from build123d import *

# Parameters (mm, degrees)
BOSS_EXTRUDE1_DEPTH            = 10
SKETCH2_W                      = 12
SKETCH2_H                      = 12.25
BOSS_EXTRUDE2_DEPTH            = 23
SKETCH4_W                      = 65
SKETCH4_H                      = 38.636969104
BOSS_EXTRUDE3_DEPTH            = 10
F_3_6_3_6_DIAMETER_HOLE1_D     = 3.6
F_3_6_3_6_DIAMETER_HOLE1_DEPTH = 10
F_3_6_3_6_DIAMETER_HOLE1_TIP   = 1.081549114
SKETCH21_W                     = 41
SKETCH21_H                     = 12.25
BOSS_EXTRUDE4_DEPTH            = 33
SKETCH23_W                     = 65
SKETCH23_H                     = 43
BOSS_EXTRUDE6_DEPTH            = 14
FILLET1_R                      = 1
F_6_6_6_6_DIAMETER_HOLE1_D     = 6.6
SKETCH28_R                     = 1.8
CUT_EXTRUDE1_DEPTH             = 44.0000001


with BuildPart() as part:
    # Sketch1 → Boss-Extrude1 (new body)
    with BuildSketch(Plane.XY):
        with BuildLine():
            Line((-6, 14.302325581), (-6, -20.697674419))
            Line((-6, -20.697674419), (6, -20.697674419))
            Line((6, -20.697674419), (6, 14.302325581))
            add(Edge.make_bspline(
                [(6, 14.302325581), (6, 18.078005618), (0, 18.078005618), (-6, 18.078005618), (-6, 14.302325581)],
                knots=[0, 0, 0, 1.570796327, 1.570796327, 3.141592654, 3.141592654, 3.141592654], degree=2, weights=[1, 0.707106781, 1, 0.707106781, 1]))
        make_face()
    boss_extrude1 = extrude(amount=BOSS_EXTRUDE1_DEPTH)

    # Sketch2 → Boss-Extrude2 (add)
    with BuildSketch(Plane.XY.offset(10)):
        with Locations((0, -14.572674419)):
            Rectangle(SKETCH2_W, SKETCH2_H)
    boss_extrude2 = extrude(amount=BOSS_EXTRUDE2_DEPTH)

    # Sketch4 → Boss-Extrude3 (add)
    with BuildSketch(Plane.XY.offset(33)):
        with Locations((-26.5, -1.379189867)):
            Rectangle(SKETCH4_W, SKETCH4_H)
    extrude(amount=BOSS_EXTRUDE3_DEPTH)

    # Mirror2: Boss-Extrude2 across plane
    add(boss_extrude2.mirror(Plane.ZY.offset(26.5)))

    # Mirror3: Boss-Extrude1 across plane
    add(boss_extrude1.mirror(Plane.ZY.offset(26.5)))

    # Ø3.6 (3.6) Diameter Hole1
    with Locations(Plane(origin=(0, 0, 0), x_dir=(-1, 0, 0), z_dir=(0, 0, -1))):
        with Locations((1.75, 7.55218084), (1.75, -2.44781916), (51.25, 8), (51.25, -2)):
            Hole(F_3_6_3_6_DIAMETER_HOLE1_D / 2, depth=F_3_6_3_6_DIAMETER_HOLE1_DEPTH)
            with Locations((0, 0, -(F_3_6_3_6_DIAMETER_HOLE1_DEPTH + F_3_6_3_6_DIAMETER_HOLE1_TIP / 2))):  # 118° drill point
                Cone(0, F_3_6_3_6_DIAMETER_HOLE1_D / 2, F_3_6_3_6_DIAMETER_HOLE1_TIP, mode=Mode.SUBTRACT)

    # Sketch21 → Boss-Extrude4 (add)
    with BuildSketch(Plane(origin=(0, 0, 33), x_dir=(-1, 0, 0), z_dir=(0, 0, -1))):
        with Locations((26.5, -14.572674419)):
            Rectangle(SKETCH21_W, SKETCH21_H)
    extrude(amount=BOSS_EXTRUDE4_DEPTH)

    # Sketch23 → Boss-Extrude6 (add)
    with BuildSketch(Plane.XZ.offset(20.697674419)):
        with Locations((-26.5, 21.5)):
            Rectangle(SKETCH23_W, SKETCH23_H)
    extrude(amount=BOSS_EXTRUDE6_DEPTH)

    # Fillet1
    fillet1_edges = [part.edges().sort_by_distance(p)[0] for p in [
        (-26.5, -8.447674419, 33),
        (0, -8.447674419, 10),
        (-26.5, 17.939294685, 33),
        (6, 17.939294685, 38),
        (-59, 17.939294685, 38),
        (-26.5, 17.939294685, 43),
        (-53, -8.447674419, 10),
        (-47, -8.447674419, 5),
        (-6, -8.447674419, 5),
    ]]
    fillet(fillet1_edges, radius=FILLET1_R)

    # Ø6.6 (6.6) Diameter Hole1 (through all)
    with Locations(Plane(origin=(0, -34.697674419, 0), x_dir=(-1, 0, 0), z_dir=(0, -1, 0))):
        with Locations((1.1, -15.5), (1.1, -25.5), (51.9, -15.5), (51.9, -25.5)):
            Hole(F_6_6_6_6_DIAMETER_HOLE1_D / 2)

    # Sketch28 → Cut-Extrude1 (cut, through all)
    with BuildSketch(Plane.XY.offset(43)):
        with Locations((-16.5, 2.553012267)):
            Circle(SKETCH28_R)
    extrude(amount=-CUT_EXTRUDE1_DEPTH, mode=Mode.SUBTRACT)


solid = part.part
Geometry: final body of the model. Coordinates: model frame, mm. A direction names the side the tool comes from. Round coordinates to 2 decimals unless told otherwise and drop trailing zeros. Loops run counter-clockwise (first coordinate to the right, second up) from the corner with the lowest first, then second, coordinate; pieces in that order, holes last.
Q1. Section B-B on z = 25.5. Return loops of the section in (x, y).
Q2. Pull-direction query (X, two-part tool) for faces 5 (the flat face through (-27, -9, 43)), 6 (the flat face through (-59, -14, 21)), 7 (the cylindrical face through (-3.719, -21.389, 17.508)); classes: released by +X, released by -X, zero draft, split by the parting line, or undercut.
Q3. Material intervals for L1, parallel to Z at x = -51.9, y = -17.5; L2, parallel to Z at x = -55.5, y = 5; L3, parallel to Y at x = -51.25, z = 2, sorted ascending.
Q4. Section C-C on y = -20. Return loops of the section in (x, z), plus the area to 3 significant figures.
Q5. Section D-D on x = -30. Return loops of the section in (y, z).
Q6. Section A-A on x = -16.5. Return loops of the section in (y, z), plus the area to 3 significant figures.
Q7. Access query for faces 1 (the flat face through (-53, 5, 10)), 2 (the cylindrical face through (-0.033, -1.907, 5.07)), 3 (the flat face through (-6, 3, 5)), 4 (the cylindrical face through (-54.519, -21.389, 27.508)). Directions: +Z, -Z, +X, -X, +Y, -Y. A direction counts if a zero-diameter tool reaches every point of the face in a straight line with its end or side. Return the directions, or none.
Q8. Pin query (flat end, axial travel): P1, Ø9.5, axis at x = -30.5, z = 16, coming from the +Y side; P2, Ø3, axis at x = -1.75, y = -2.45, coming from the -Z side; P3, Ø5.5, axis at x = -51.9, z = 15.5, coming from the -Y side; P4, Ø9, axis at x = -41, z = 37, coming from the +Y side. Return the tip coordinate at first contact, or that it passes through.
Evaluation:
1. outline: (-59, -34.7) - (-55.2, -34.7) - (-55.2, -8.45) - (-59, -8.45) - close; (-48.6, -34.7) - (-4.4, -34.7) - (-4.4, -8.45) - (-48.6, -8.45) - close; (2.2, -34.7) - (6, -34.7) - (6, -8.45) - (2.2, -8.45) - close
2. face 5: zero draft
2. face 6: released by -X
2. face 7: undercut
3. L1: z = 0 to 12.2, 18.8 to 22.2, 28.8 to 43
3. L2: z = 0 to 10, 33 to 43
3. L3: y = -34.7 to -3.8, -0.2 to 6.2, 9.8 to 17.91
4. outline: (-59, 0) - (6, 0) - (6, 43) - (-59, 43) - close; hole circle Ø6.6 at (-51.9, 15.5); hole circle Ø6.6 at (-51.9, 25.5); hole circle Ø6.6 at (-1.1, 15.5); hole circle Ø6.6 at (-1.1, 25.5)
4. area: 2,660 mm2
5. outline: (-34.7, 0) - (-8.45, 0) - (-8.45, 32) arc R1 cw to (-7.45, 33) - (16.94, 33) arc R1 ccw to (17.94, 34) - (17.94, 42) arc R1 ccw to (16.94, 43) - (-34.7, 43) - close
6. outline: (-34.7, 0) - (-8.45, 0) - (-8.45, 32) arc R1 cw to (-7.45, 33) - (0.75, 33) - (0.75, 43) - (-34.7, 43) - close; (4.35, 33) - (16.94, 33) arc R1 ccw to (17.94, 34) - (17.94, 42) arc R1 ccw to (16.94, 43) - (4.35, 43) - close
6. area: 1,360 mm2
7. face 1: +X, -X, +Y
7. face 2: -Z
7. face 3: -Z, +Y
7. face 4: +Y, -Y
8. P1: stops at y = -8.45
8. P2: stops at z = 33
8. P3: passes through
8. P4: stops at y = 17.94
